Autodesk Inventor part; units mm, degrees
ref_plane "YZ Plane" through (0, 0, 0) normal (1, 0, 0) x (0, 1, 0)
ref_plane "XZ Plane" through (0, 0, 0) normal (0, 1, 0) x (-1, 0, 0)
ref_plane "XY Plane" through (0, 0, 0) normal (0, 0, 1) x (1, 0, 0)
sketch "Sketch1" plane through (0, 0, 0) normal (0, 0, 1) x (1, 0, 0)
  line L0 (0, 0) -> (0, -59.4) construction
  line L1 (0, -59.4) -> (7.5, -59.4)
  line L2 (7.5, -59.4) -> (7.5, -66.4)
  line L3 (7.5, -66.4) -> (5, -66.4)
  line L4 (5, -66.4) -> (5, -63.4)
  line L5 (5, -63.4) -> (0, -63.4)
  line L6 (0, -63.4) -> (0, -59.4)
  line L7 (0, 0) -> (7.5, 0) construction
  line L8 (7.5, 0) -> (7.5, -59.4) construction
  line L9 (7.5, -59.4) -> (7.5, -66.4)
  dimension "d0" = 63.4
  dimension "d1" = 4
  dimension "d2" = 2.5
  dimension "d3" = 3
  dimension "d4" = 5
revolve "Revolution1" add sketch "Sketch1" angle 360 about axis through (0, 0, 0) along (1, 0, 0)
sketch "Sketch2" plane through (0, 0, 0) normal (-1, 0, 0) x (0, 0, 1)
  line L0 (0, 0) -> (0, 55.6716) construction
  line L1 (0, 0) -> (-59.868, 0) construction
  line L2 (0, 0) -> (-47.9174, -40.2075) construction
  line L3 (0, 0) -> (-42.8366, 35.9442) construction
  circle A0 centre (-45.8861, 38.503) radius 3.5 construction
  circle A1 centre (-59.9, 0) radius 3.5 construction
  circle A2 centre (-45.8861, -38.503) radius 3.5 construction
  circle A3 centre (-45.8861, 38.503) radius 1.75
  circle A4 centre (-45.8861, 38.503) radius 4.5
  circle A5 centre (-59.9, 0) radius 4.5
  circle A6 centre (-59.9, 0) radius 1.75
  circle A7 centre (-45.8861, -38.503) radius 1.75
  circle A8 centre (-45.8861, -38.503) radius 4.5
  circle A9 centre (0, 0) radius 63.4
  circle A10 centre (45.8861, 38.503) radius 1.75
  circle A11 centre (45.8861, 38.503) radius 3.5 construction
  circle A12 centre (45.8861, 38.503) radius 4.5
  circle A13 centre (59.9, 0) radius 1.75
  circle A14 centre (59.9, 0) radius 4.5
  circle A15 centre (59.9, 0) radius 3.5 construction
  circle A16 centre (45.8861, -38.503) radius 3.5 construction
  circle A17 centre (45.8861, -38.503) radius 1.75
  circle A18 centre (45.8861, -38.503) radius 4.5
  point P0 (-24.75, 53.9981)
  point P1 (-57.3891, -15.325)
  point P2 (57.3891, -15.325)
  point P3 (42.8366, 35.9442)
  point P4 (59.868, 0)
  point P5 (47.9174, -40.2075)
  point P6 (-46.6461, 42.9383)
  point P7 (-50.386, 38.4813)
  point P8 (-63.3332, 2.9091)
  point P9 (-63.3332, -2.9091)
  point P10 (-50.386, -38.4813)
  point P11 (-46.6461, -42.9383)
  point P12 (46.6461, 42.9383)
  point P13 (50.386, 38.4813)
  point P14 (63.3332, 2.9091)
  point P15 (63.3332, -2.9091)
  point P16 (50.386, -38.4813)
  point P17 (46.6461, -42.9383)
  dimension "d9" = 40
  dimension "d10" = 40
  dimension "d11" = 7
  dimension "d12" = 9
  dimension "d13" = 3.5
extrude "Extrusion1" add sketch "Sketch2" against normal up to surface (7.5 mm away) contours A4 A9 | A9 A12 | A5 A9 | A9 A14 | A8 A9 | A9 A18 picked at (-46.8937, 41.5565) picked at (46.8937, 41.5565) picked at (-62.6452, -1.6799) picked at (62.3698, 2.2508) picked at (-46.8937, -41.5565) picked at (46.8937, -41.5565)
extrude "Extrusion2" cut sketch "Sketch2" against normal through all contours A3 | A6 | A7 | A10 | A13 | A17
sketch "Sketch3" plane through (7.5, 0, 0) normal (1, 0, 0) x (0, 0, -1)
  circle A0 centre (-45.8861, 38.503) radius 1.75
  circle A1 centre (-45.8861, 38.503) radius 3
  circle A2 centre (-59.9, 0) radius 1.75
  circle A3 centre (-59.9, 0) radius 3
  circle A4 centre (-45.8861, -38.503) radius 1.75
  circle A5 centre (-45.8861, -38.503) radius 3
  circle A6 centre (45.8861, -38.503) radius 1.75
  circle A7 centre (45.8861, -38.503) radius 3
  circle A8 centre (59.9, 0) radius 1.75
  circle A9 centre (59.9, 0) radius 3
  circle A10 centre (45.8861, 38.503) radius 1.75
  circle A11 centre (45.8861, 38.503) radius 3
  point P0 (0, 0)
  dimension "d18" = 6
extrude "Extrusion3" cut sketch "Sketch3" against normal blind 3 contours A0 | A1 | A2 | A3 | A4 | A5 | A6 | A7 | A8 | A9 | A10 | A11
equation "\"d10\" = d9"
properties part number "SwivelMountClamp"
The model under review builds one solid part; all positions refer to its coordinate system, in mm. A direction names the side the tool comes from. Coordinates: 2 decimals unless noted, no trailing zeros. Loops run counter-clockwise (first coordinate to the right, second up) from the corner with the lowest first, then second, coordinate; pieces in that order, holes last. Notation, with made-up numbers: (-16, 9.25) -> (38, 9.25) arc R26 ccw to (38, 47.25) -> close; hole circle Ø11 at (-10.5, 88.25). An arc over 180 degrees is marked (long way). Use a Markdown table: item, result. Add a question column.
1. Add section C-C on y = 22. Write out the cut boundary in (x, z).
2. Add section B-B on z = -16. Write out the cut boundary in (x, y).
3. Machinability: for faces 1 (the face through (0, -37, -43)), 2 (the face through (6.02, 0.9, -62.76)), 3 (the face through (3.7, -0.1, -55.4)), 4 (the face through (2.465, -60.472, 19.044)), which of the approach directions +Z, -Z, +X, -X, +Y, -Y give a long, thin tool a straight path to every point of the face, cutting with its end or side? Answer none if there is none.
4. Add section D-D on x = 2.75. Write out the cut boundary in (y, z).
5. Add section A-A on y = 0. Write out the cut boundary in (x, z), plus the area to 3 significant figures.
6. Draft analysis for pull direction Z (two halves, no side actions). For faces 5 (the face through (3.7, -35.54, 42.5)), 6 (the face through (2.218, 36.858, -46.483)), 7 (the face through (7.5, 35, 44)), 8 (the face through (6.23, 14.39, -64.82)), state which applies: pulls with the +Z half, pulls with the -Z half, needs draft (parallel to the pull), parting line crosses it, or undercut.
7. To check wall thickness, follow line 1 (Z direction, x = 3.5, y = 1); line 2 (Z direction, x = 4.25, y = 9); line 3 (Y direction, x = 6, z = 16.5). State the ranges of each line that lie inside material, in increasing order.
8. Clearance check with flat-ended pins moving along their axes: pin 1 Ø3 at (x, z) = (4, -14.5) entering from +Y; pin 2 Ø2 at (x, z) = (5.5, -16.5) entering from -Y; pin 3 Ø1.8 at (y, z) = (-39.5, -47) entering from +X. State where each tip first meets the part, or that it passes through.
Returned:
| question | item | result |
|---|---|---|
| 1 | outline | (0, -59.46) -> (5, -59.46) -> (5, -62.65) -> (7.5, -62.65) -> (7.5, -55.18) -> (0, -55.18) -> close; (0, 55.18) -> (7.5, 55.18) -> (7.5, 62.65) -> (5, 62.65) -> (5, 59.46) -> (0, 59.46) -> close |
| 2 | outline | (0, -61.35) -> (5, -61.35) -> (5, -64.44) -> (7.5, -64.44) -> (7.5, -57.2) -> (0, -57.2) -> close; (0, 57.2) -> (7.5, 57.2) -> (7.5, 64.44) -> (5, 64.44) -> (5, 61.35) -> (0, 61.35) -> close |
| 3 | face 1 | +Z, -Z, -X, +Y, -Y |
| 3 | face 2 | +X |
| 3 | face 3 | +X, -X |
| 3 | face 4 | -X |
| 4 | outline | circle Ø126.8 at (0, 0); hole (-41.48, -42.51) arc R4.5 cw to (-34.67, -48.24) arc R59.4 ccw to (-4.45, -59.23) arc R4.5 cw to (4.45, -59.23) arc R59.4 ccw to (34.67, -48.24) arc R4.5 cw to (41.48, -42.51) arc R59.4 ccw to (41.48, 42.51) arc R4.5 cw to (34.67, 48.24) arc R59.4 ccw to (4.45, 59.23) arc R4.5 cw to (-4.45, 59.23) arc R59.4 ccw to (-34.67, 48.24) arc R4.5 cw to (-41.48, 42.51) arc R59.4 ccw to start; hole circle Ø3.5 at (-38.5, -45.89); hole circle Ø3.5 at (-38.5, 45.89); hole circle Ø3.5 at (0, -59.9); hole circle Ø3.5 at (0, 59.9); hole circle Ø3.5 at (38.5, -45.89); hole circle Ø3.5 at (38.5, 45.89) |
| 5 | outline | (0, -63.4) -> (5, -63.4) -> (5, -66.4) -> (7.5, -66.4) -> (7.5, -62.9) -> (4.5, -62.9) -> (4.5, -61.65) -> (0, -61.65) -> close; (0, -58.15) -> (4.5, -58.15) -> (4.5, -56.9) -> (7.5, -56.9) -> (7.5, -55.4) -> (0, -55.4) -> close; (0, 55.4) -> (7.5, 55.4) -> (7.5, 56.9) -> (4.5, 56.9) -> (4.5, 58.15) -> (0, 58.15) -> close; (0, 61.65) -> (4.5, 61.65) -> (4.5, 62.9) -> (7.5, 62.9) -> (7.5, 66.4) -> (5, 66.4) -> (5, 63.4) -> (0, 63.4) -> close |
| 5 | area | 67.5 mm² |
| 6 | face 5 | undercut |
| 6 | face 6 | undercut |
| 6 | face 7 | needs draft |
| 6 | face 8 | parting line crosses it |
| 7 | line 1 | z = -63.39 to -61.34, -58.46 to -55.51, 55.51 to 58.46, 61.34 to 63.39 |
| 7 | line 2 | z = -62.76 to -58.71, 58.71 to 62.76 |
| 7 | line 3 | y = -64.32 to -57.06, 57.06 to 64.32 |
| 8 | pin 1 | stops at y = 65.04 |
| 8 | pin 2 | stops at y = -64.57 |
| 8 | pin 3 | stops at x = 4.5 |
